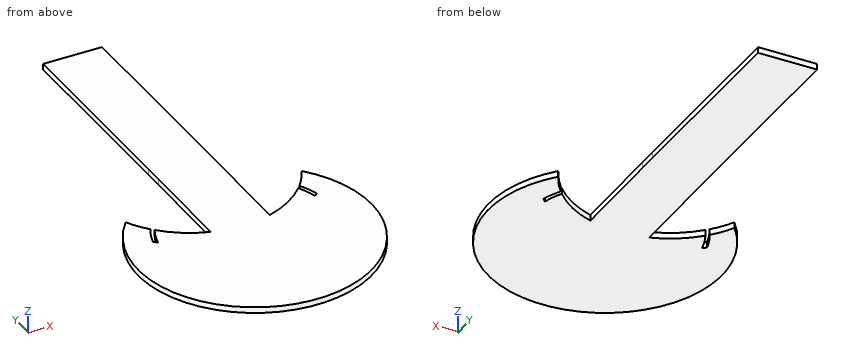
from build123d import *

# Parameters (mm, degrees)
F0_W     = 60
F0_H     = 200
F1_DEPTH = 6


# Not quite as in the source:
# - the program builds the solid bodies; features that only make, move or delete a surface that nothing else refers to are left out


with BuildPart() as f1:
    # F0 (on Top) → F1 (new body)
    with BuildSketch(Plane.XY):
        with Locations((4.8876879096, 35.2179194741)):
            Rectangle(F0_W, F0_H)
        with BuildLine():
            ThreePointArc((-79.4584430704, -175.2136584167), (-76.086405566, -164.9666401832), (-71.4764851469, -155.2136584167))
            ThreePointArc((-71.4764851469, -155.2136584167), (-79.1565485083, -145.3205641479), (-85.5490516624, -134.5505784994))
            ThreePointArc((-85.5490516624, -134.5505784994), (6.1468085688, -329.3233337338), (94.4628409087, -132.9949471034))
            ThreePointArc((94.4628409087, -132.9949471034), (88.2574232589, -143.8738017875), (80.7494829473, -153.8981481364))
            ThreePointArc((80.7494829473, -153.8981481364), (85.2254366965, -162.8589485125), (88.6456429035, -172.2734211397))
            ThreePointArc((88.6456429035, -172.2734211397), (75.2367314586, -249.2062042963), (5.6459887203, -284.6403764396))
            ThreePointArc((5.6459887203, -284.6403764396), (-63.9155377146, -250.9329661403), (-79.4584430704, -175.2136584167))
        make_face()
        with BuildLine():
            ThreePointArc((4.8876879096, -189.3289751767), (-10.6634233248, -188.2490297182), (-25.8614792361, -184.7816907769))
            ThreePointArc((-25.8614792361, -184.7816907769), (-48.9823809676, -174.2243385437), (-68.7229965841, -158.2136584167))
            ThreePointArc((-68.7229965841, -158.2136584167), (-72.9335538665, -167.9839691049), (-75.8560904631, -178.2136584167))
            ThreePointArc((-75.8560904631, -178.2136584167), (-59.2361153237, -247.9542245013), (5.5975931326, -278.5574984969))
            Line((5.5975931326, -278.5574984969), (4.8876879096, -189.3289751767))
        make_face()
        with BuildLine():
            ThreePointArc((78.0917461365, -156.8981481364), (57.9442467877, -173.7054474984), (34.1385207639, -184.7369682609))
            ThreePointArc((34.1385207639, -184.7369682609), (19.6828166371, -188.1140297879), (4.8876879096, -189.3289751767))
            Line((4.8876879096, -189.3289751767), (5.5975931326, -278.5574984969))
            ThreePointArc((5.5975931326, -278.5574984969), (70.4913174106, -246.4384867175), (85.2871903638, -175.5589515052))
            ThreePointArc((85.2871903638, -175.5589515052), (82.255170922, -166.010419768), (78.0917461365, -156.8981481364))
        make_face()
        with BuildLine():
            ThreePointArc((5.5975931326, -278.5574984969), (-59.2361153237, -247.9542245013), (-75.8560904631, -178.2136584167))
            Line((-75.8560904631, -178.2136584167), (-79.4584430704, -175.2136584167))
            ThreePointArc((-79.4584430704, -175.2136584167), (-63.9155377146, -250.9329661403), (5.6459887203, -284.6403764396))
            Line((5.6459887203, -284.6403764396), (5.5975931326, -278.5574984969))
        make_face()
        with BuildLine():
            ThreePointArc((85.2871903638, -175.5589515052), (70.4913174106, -246.4384867175), (5.5975931326, -278.5574984969))
            Line((5.5975931326, -278.5574984969), (5.6459887203, -284.6403764396))
            ThreePointArc((5.6459887203, -284.6403764396), (75.2367314586, -249.2062042963), (88.6456429035, -172.2734211397))
            Line((88.6456429035, -172.2734211397), (85.2871903638, -175.5589515052))
        make_face()
        with BuildLine():
            Line((34.7627821954, -84.7816907769), (-25.2371712536, -84.7816907769))
            Line((-25.2371712536, -84.7816907769), (-25.8614792361, -184.7816907769))
            ThreePointArc((-25.8614792361, -184.7816907769), (-10.6634233248, -188.2490297182), (4.8876879096, -189.3289751767))
            ThreePointArc((4.8876879096, -189.3289751767), (19.6828166371, -188.1140297879), (34.1385207639, -184.7369682609))
            Line((34.1385207639, -184.7369682609), (34.7627821954, -84.7816907769))
        make_face()
        Polygon((34.8876879096, -64.7820805259), (-25.1123120904, -64.7820805259), (-25.2371712536, -84.7816907769), (34.7627821954, -84.7816907769), align=None)
    extrude(amount=F1_DEPTH)


solid = f1.part
Could you check a few things on this model? Use its own coordinates, in mm. Give positions to 0.01 mm unless a question says otherwise; leave off trailing zeros. Loops run counter-clockwise (first coordinate to the right, second up) from the corner with the lowest first, then second, coordinate; pieces in that order, holes last. Notation, with made-up numbers: M -6.75,-26 L 7.25,-26 A22 ccw 7.25,-13 Z; hole C 18,84 d7. An arc over 180 degrees is marked long. Answer as a JSON object with one key per item and string values.
Q1. For P1, Ø1.8, axis at y = 75, z = 2.5, coming from the -X side; P2, Ø2, axis at x = 39, z = 1.5, coming from the +Y side; P3, Ø1.5, axis at y = 22.5, z = 5.5, coming from the +X side, each with a flat end and sliding along its axis, tell me the tip position at first contact or that it passes through.
Values found:
{"P1": "stops at x = -25.11", "P2": "stops at y = -182.7", "P3": "stops at x = 34.89"}
Q2. If I drill on probe 1 along X at (y, z) = (6, 3.8); probe 2 along X at (y, z) = (-150, 3.95); probe 3 along Y at (x, z) = (19, 1.3), over which ranges is the centre line in solid material (lowest first)? Write a range as [from, to].
Values found:
{"probe 1": "x = [-25.11, 34.89]", "probe 2": "x = [-96.56, -75.77], [-25.64, 34.36], [83.9, 106.81]", "probe 3": "y = [-328.51, 135.22]"}
Q3. Suppose I cut it at B-B, the plane y = -3.5. List the corners of the cut face in (x, z) for me.
Values found:
{"outline": "M -25.11,0 L 34.89,0 L 34.89,6 L -25.11,6 Z"}
Q4. Suppose I cut it at C-C, the plane x = -32. List the corners of the cut face in (y, z) for me.
Values found:
{"outline": "M -323.36,0 L -182.65,0 L -182.65,6 L -323.36,6 Z"}
Q5. Suppose I cut it at A-A, the plane z = 2.85. List the corners of the cut face in (x, y) for me.
Values found:
{"outline": "M -85.55,-134.55 A118.49 ccw long 94.46,-132.99 A100.69 cw 80.75,-153.9 A87.31 cw 88.65,-172.27 L 85.29,-175.56 A82.77 ccw 78.09,-156.9 A100.69 cw 34.14,-184.74 L 34.89,-64.78 L 34.89,135.22 L -25.11,135.22 L -25.11,-64.78 L -25.86,-184.78 A100.69 cw -68.72,-158.21 A82.77 ccw -75.86,-178.21 L -79.46,-175.21 A87.31 cw -71.48,-155.21 A100.69 cw Z"}
